Check sheet for the drawn part. Datum: minimum x, y, z corner. Units: mm. Give positions to 0.01 mm unless a question says otherwise; leave off trailing zeros. Write each loop counter-clockwise with the first axis right and the second up, starting at its lowest first coordinate (ties: lowest second). Pieces come first, ordered by that corner, then holes. Notation, with made-up numbers: (10.5, -28.75) -> (21.5, -28.75) arc R17 cw to (21.5, 1.25) -> close; hole circle Ø10 at (-33, -21.5). An arc over 180 degrees is marked (long way). Write item = value, one per line. Start each with the question number.
1. Cross-section at D-D, the plane y = 16. Record the cut outline in (x, z).
2. Thickness scan on line 1 along Y through (x, z) = (2.5, 0.5); line 2 along X through (y, z) = (3.25, 3.75); line 3 along X through (y, z) = (26, 4.25). Record the ranges inside material, lowest first.
3. Cross-section at A-A, the plane x = 3.25. Record the cut outline in (y, z), plus the area to 3 significant figures.
4. Mould release check, pull along Y, two halves, no side actions. Record for the marked faces 1, 2 and 3: pulls with the +Y half, pulls with the -Y half, needs draft (parallel to the pull), parting line crosses it, or undercut.
5. Depth check by flat-ended pin: P1, Ø1, axis at y = 4, z = 2.5, coming from the -X side; P2, Ø3, axis at x = 3.25, y = 4, coming from the +Z side; P3, Ø2, axis at x = 3.25, y = 26, coming from the -Z side. Enter the tip coordinate at first touch or a pass-through.
6. Cross-section at C-C, the plane y = 4. Record the cut outline in (x, z), plus the area to 3 significant figures.
7. Cross-section at B-B, the plane z = 3.25. Record the cut outline in (x, y), plus the area to 3 significant figures.
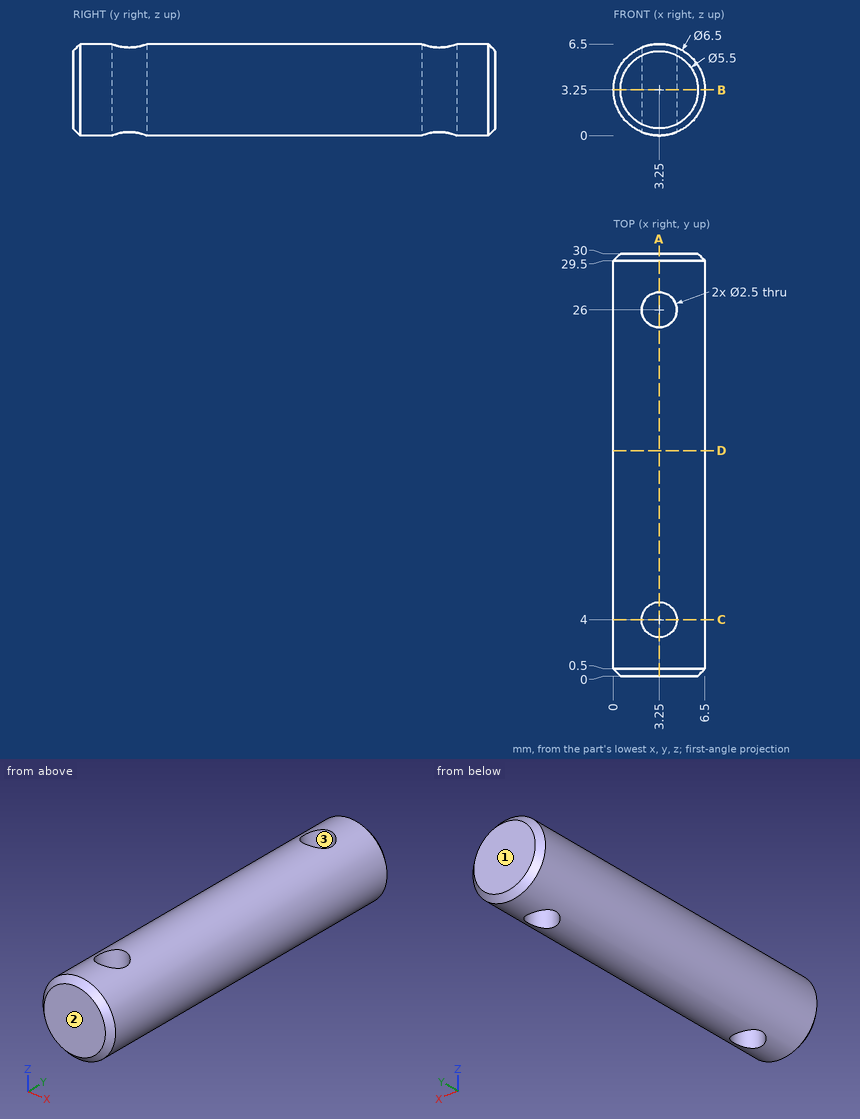
Answers:
q1.outline = circle Ø6.5 at (3.25, 3.25)
q2.line_1 = 0.1 to 3, 5 to 25, 27 to 29.9
q2.line_2 = 0.04 to 2.25, 4.25 to 6.46
q2.line_3 = 0.16 to 2, 4.5 to 6.34
q3.outline = (0, 0.5) -> (0.5, 0) -> (2.75, 0) -> (2.75, 6.5) -> (0.5, 6.5) -> (0, 6) -> close; (5.25, 0) -> (24.75, 0) -> (24.75, 6.5) -> (5.25, 6.5) -> close; (27.25, 0) -> (29.5, 0) -> (30, 0.5) -> (30, 6) -> (29.5, 6.5) -> (27.25, 6.5) -> close
q3.area = 162 mm^2
q4.face_1 = pulls with the +Y half
q4.face_2 = pulls with the -Y half
q4.face_3 = undercut
q5.P1 = 0.01
q5.P2 = 6.5
q5.P3 = through
q6.outline = (2, 0.25) -> (2, 6.25) arc R3.25 ccw to start; (4.5, 0.25) arc R3.25 ccw to (4.5, 6.25) -> close
q6.area = 17.3 mm^2
q7.outline = (0, 0.5) -> (0.5, 0) -> (6, 0) -> (6.5, 0.5) -> (6.5, 29.5) -> (6, 30) -> (0.5, 30) -> (0, 29.5) -> close; hole circle Ø2.5 at (3.25, 4); hole circle Ø2.5 at (3.25, 26)
q7.area = 185 mm^2
